Job drawing, mm, ordinate dimensions from the low corner. One solid piece. A direction names the side the tool comes from. Give positions to 0.01 mm unless a question says otherwise; leave off trailing zeros. Write each loop counter-clockwise with the first axis right and the second up, starting at its lowest first coordinate (ties: lowest second). Pieces come first, ordered by that corner, then holes. Notation, with made-up numbers: (40, 66) - (65, 66) arc R34 ccw to (65, 99) - close; hole circle Ø9 at (32.5, -11). An arc over 180 degrees is marked (long way). Answer as a JSON object with one key per item and string values.
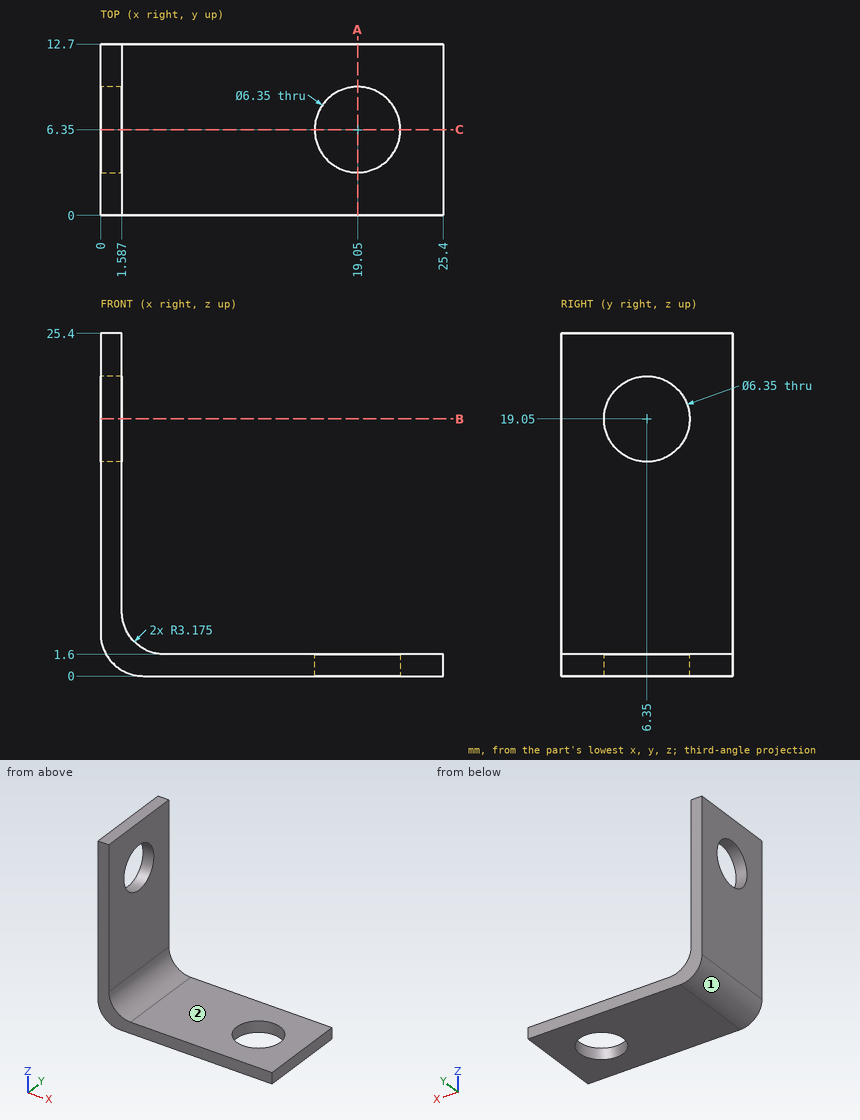
Item 1: Cut at C-C (y = 6.35). State how many separate pieces and enclosed holes the cut face has.
Entries:
{"separate pieces": "3", "enclosed holes": "0"}
Item 2: Cut at B-B (z = 19.05). Give the cut face in (x, y) (1 decimal).
Entries:
{"outline": "(0, 0) - (1.6, 0) - (1.6, 3.2) - (0, 3.2) - close; (0, 9.5) - (1.6, 9.5) - (1.6, 12.7) - (0, 12.7) - close"}
Item 3: Cut at A-A (x = 19.05). Give the cut face in (y, z) (1 decimal).
Entries:
{"outline": "(0, 0) - (3.2, 0) - (3.2, 1.6) - (0, 1.6) - close; (9.5, 0) - (12.7, 0) - (12.7, 1.6) - (9.5, 1.6) - close"}
Item 4: Flat gauge pins, fed straight in: P1, Ø1.5, axis at y = 7.5, z = 21.5, coming from the +X side; P2, Ø6.5, axis at x = 10.5, y = 5.5, coming from the +Z side. Where does each tip first touch, or does it go through?
Entries:
{"P1": "x = 1.59", "P2": "z = 1.6"}
Item 5: Probe line 1 (Y direction, x = 19.05, z = 0.8) (1 decimal); line 2 (Z direction, x = 6, y = 8); line 3 (Z direction, x = 0.5, y = 6.35) (1 decimal). List the from-to ranges inside material, lowest first. Write a range as from..to.
Entries:
{"line 1": "0..3.2, 9.5..12.7", "line 2": "0..1.6", "line 3": "1.5..15.9, 22.2..25.4"}
Item 6: Which spindle directions (+Z, -Z, +X, -X, +Y, -Y) get a long thin tool onto all of the face, cutting with end or side? Do the marked faces 1 and 2. Say none if no direction does.
Entries:
{"face 1": "-Z, -X, +Y, -Y", "face 2": "+Z, +X, +Y, -Y"}
